Check sheet for the modelled part. Datum: model origin and axes. Units: mm. Face numbers are marked on the shaded views. A direction names the side the tool comes from. Give positions to 0.01 mm unless a question says otherwise; leave off trailing zeros. Write each loop counter-clockwise with the first axis right and the second up, starting at its lowest first coordinate (ties: lowest second). Pieces come first, ordered by that corner, then holes.
from build123d import *

# Parameters (mm, degrees)
F0_R     = 2
F1_DEPTH = 15
F2_R     = 2.75
F3_DEPTH = 15.001


with BuildPart() as f1:
    # F0 (on Top) → F1 (new body)
    with BuildSketch(Plane.XY):
        with BuildLine():
            ThreePointArc((7.292976, 1.75), (4.643544, 5.889609), (0, 7.5))
            ThreePointArc((0, 7.5), (-7.5, 0), (0, -7.5))
            ThreePointArc((0, -7.5), (4.643544, -5.889609), (7.292976, -1.75))
            Line((7.292976, -1.75), (3.031089, -1.75))
            ThreePointArc((3.031089, -1.75), (-3.5, 0), (3.031089, 1.75))
            Line((3.031089, 1.75), (7.292976, 1.75))
        make_face()
        with BuildLine():
            ThreePointArc((30, -7.5), (22.5, 0), (30, 7.5))
            Line((30, 7.5), (0, 7.5))
            ThreePointArc((0, 7.5), (4.643544, 5.889609), (7.292976, 1.75))
            Line((7.292976, 1.75), (20.031089, 1.75))
            ThreePointArc((20.031089, 1.75), (21.781089, 0), (20.031089, -1.75))
            Line((20.031089, -1.75), (7.292976, -1.75))
            ThreePointArc((7.292976, -1.75), (4.643544, -5.889609), (0, -7.5))
            Line((0, -7.5), (30, -7.5))
        make_face()
        with BuildLine():
            ThreePointArc((30, -7.5), (35.303301, -5.303301), (37.5, 0))
            ThreePointArc((37.5, 0), (35.303301, 5.303301), (30, 7.5))
            ThreePointArc((30, 7.5), (22.5, 0), (30, -7.5))
        make_face()
        with Locations((30, 0)):
            Circle(F0_R, mode=Mode.SUBTRACT)
    extrude(amount=F1_DEPTH)

    # F2 (on face) → F3 (cut, through all)
    with BuildSketch(Plane.XZ.offset(7.5)):
        with Locations((11.531089, 7.5)):
            Circle(F2_R)
    extrude(amount=-F3_DEPTH, mode=Mode.SUBTRACT)


solid = f1.part
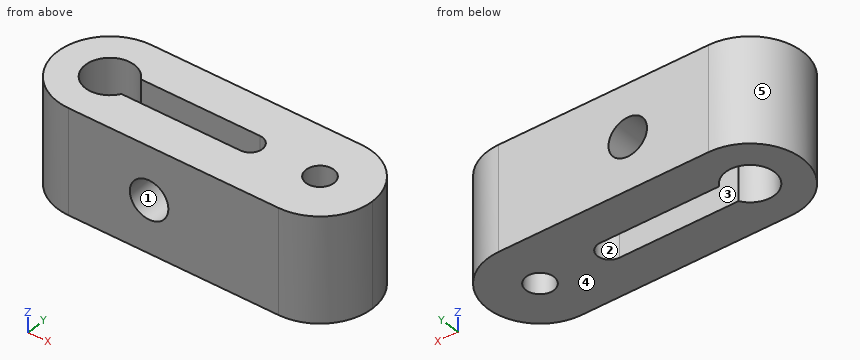
1) Sectioned sample at C-C on y = -0.5. Record the boundary of the cut face in (x, z).
2) Scan lines: L1, parallel to Y at x = 18.5, z = 9.75; L2, parallel to Y at x = -1.5, z = 3.75; L3, parallel to X at y = -0.25, z = 4.5. Record each from-to range of solid material in increasing order.
3) Sectioned sample at B-B on x = 16.5. Record the boundary of the cut face in (y, z).
4) Sectioned sample at A-A on z = 7.5. Record the boundary of the cut face in (x, y), then the cut area to 3 significant figures.
5) Draft check along X on the marked faces 3, 4 and 5. Enter one of: +X half, -X half, draft (parallel to the pull), parting line (faces both ways), or undercut.
6) Sectioned sample at D-D on y = -3. Record the boundary of the cut face in (x, z), then the cut area to 3 significant figures.
7) Gauge pin test, flat end, axial feed: pin 1 (5 mm diameter, centred on x = 11.53, z = 7.5, fed in from +Y). Record the tip position at first contact, or that the pin passes through.
8) Access from +Z, -Z, +X, -X, +Y, -Y to the whole of each face (thin tool, end or side, straight path). Record for the marked faces 1 and 2.
Answers below:
1. outline: (-7.48, 0) - (-3.46, 0) - (-3.46, 15) - (-7.48, 15) - close; (21.71, 0) - (28.06, 0) - (28.06, 15) - (21.71, 15) - close; (31.94, 0) - (37.48, 0) - (37.48, 15) - (31.94, 15) - close
2. L1: y = -7.5 to -1.75, 1.75 to 7.5
2. L2: y = -7.35 to -3.16, 3.16 to 7.35
2. L3: x = -7.5 to -3.49, 21.76 to 28.02, 31.98 to 37.5
3. outline: (-7.5, 0) - (-1.75, 0) - (-1.75, 15) - (-7.5, 15) - close; (1.75, 0) - (7.5, 0) - (7.5, 15) - (1.75, 15) - close
4. outline: (0, -7.5) - (8.78, -7.5) - (8.78, -1.75) - (3.03, -1.75) arc R3.5 cw (long way) to (3.03, 1.75) - (8.78, 1.75) - (8.78, 7.5) - (0, 7.5) arc R7.5 ccw to start; (14.28, -7.5) - (30, -7.5) arc R7.5 ccw to (30, 7.5) - (14.28, 7.5) - (14.28, 1.75) - (20.03, 1.75) arc R1.75 cw to (20.03, -1.75) - (14.28, -1.75) - close; hole circle Ø4 at (30, 0)
4. area: 449 mm2
5. face 3: undercut
5. face 4: draft
5. face 5: -X half
6. outline: (-6.87, 0) - (-1.8, 0) - (-1.8, 15) - (-6.87, 15) - close; (1.8, 0) - (36.87, 0) - (36.87, 15) - (1.8, 15) - close; hole circle Ø5.5 at (11.53, 7.5)
6. area: 578 mm2
7. pin 1: passes through
8. face 1: +Y, -Y
8. face 2: +Z, -Z
